Solid Edge part; units mm, degrees
sketch "Sketch1" plane through (0, 0, 0) normal (0, 0, 1) x (1, 0, 0)
  line L0 (-10, -20) -> (10, -20)
  line L1 (10, -20) -> (10, 20)
  line L2 (10, 20) -> (-10, 20)
  line L3 (-10, 20) -> (-10, -20)
extrude "Protrusion1" add sketch "Sketch1" along normal blind 62
sketch "Sketch2" plane through (-10, 0, 31) normal (-1, 0, 0) x (0, -1, 0)
  line L0 (20, -31) -> (20, -1)
  line L1 (20, -1) -> (1, -1)
  line L2 (1, -1) -> (1, -31)
  line L3 (1, -31) -> (20, -31)
  dimension "D1" = 1
extrude "Cutout1" cut sketch "Sketch2" along normal through all and the other way through all
sketch "Sketch3" plane through (-10, 0, 31) normal (-1, 0, 0) x (0, -1, 0)
  line L0 (-20, 31) -> (-8, 31)
  line L1 (-20, -7) -> (-8, 31)
  line L2 (-20, 31) -> (-20, -7)
extrude "Cutout2" cut sketch "Sketch3" along normal through all and the other way through all
hole "Hole1" at (7, 4, 62) direction (0, 0, -1) diameter 3 depth 9 tip angle 118
hole "Hole2" at (-7, 4, 62) direction (0, 0, -1) diameter 3 depth 9 tip angle 118
hole "Hole3" at (-7, -17, 62) direction (0, 0, -1) diameter 3 depth 9 tip angle 118
hole "Hole4" at (7, -17, 62) direction (0, 0, -1) diameter 3 depth 9 tip angle 118
sketch "Sketch4" plane through (0, -6, 62) normal (0, 0, 1) x (1, 0, 0)
  circle A0 centre (0, -4) radius 7
extrude "Cutout3" cut sketch "Sketch4" along normal up to next and the other way up to next
sketch "Sketch5" plane through (0, -20, 46) normal (0, -1, 0) x (1, 0, 0)
  circle A0 centre (-3, -1) radius 1.6
  circle A1 centre (3, -1) radius 1.6
  dimension "D1" = 3
extrude "Cutout4" cut sketch "Sketch5" along normal up to next and the other way up to next
sketch "Sketch6" plane through (0, 20, 12) normal (0, 1, 0) x (0, 0, -1)
  circle A0 centre (2, 0) radius 4
  dimension "D1" = 2
extrude "Cutout5" cut sketch "Sketch6" along normal up to next and the other way up to next
chamfer "Fase_an_schaft" distance 1 angle 45 1 edges at (0, 20, 14)
sketch "Sketch7" plane through (0, 9.5, 0) normal (0, 0, -1) x (1, 0, 0)
  circle A0 centre (0, 5.5) radius 2
extrude "Cutout6" cut sketch "Sketch7" along normal up to next and the other way up to next
hole "auslass_oben" at (0, 4, 62) direction (0, 0, -1) diameter 2.5 end up to next counterbore diameter 4 counterbore depth 30
sketch "Sketch8" plane through (-10, 0, 31) normal (-1, 0, 0) x (0, 0, -1)
  circle A0 centre (11, -12) radius 2.3428
extrude "Cutout7" cut sketch "Sketch8" along normal up to next and the other way up to next
sketch "Sketch9" plane through (0, 9.5, 0) normal (0, 0, -1) x (0, -1, 0)
  circle A0 centre (-2.5, 0) radius 2
extrude "auslassloch_hinten" cut sketch "Sketch9" against normal blind 20
sketch "Sketch10" plane through (0, -6, 62) normal (0, 0, 1) x (0, -1, 0)
  line L0 (-10, -2) -> (1.0843, -2)
  line L1 (1.0843, -2) -> (1.0843, 2)
  line L2 (1.0843, 2) -> (-10, 2)
  line L3 (-10, 2) -> (-10, -2)
  dimension "D1" = 1.0843
extrude "fräsung_oben" cut sketch "Sketch10" against normal blind 2
CAD build for the part. Positions are in the model's coordinates, mm. A direction names the side the tool comes from. Round coordinates to 2 decimals unless told otherwise and drop trailing zeros. Order: outer loops, then holes, each group sorted by start corner. A loop starts at its lowest first (then second) coordinate and runs counter-clockwise, first axis right, second up.
Item 1: Saw through at C-C on y = 12. Write the cut outline in (x, z).
Item 2: Tool access for faces 4 (the face through (-0.601, 10.092, 16.085)), 5 (the face through (-2, -17, 30)), 6 (the face through (-5.536, 4.325, 57.437)), 7 (the face through (-5.555, -14.259, 46.224)): list every direction of +Z, -Z, +X, -X, +Y, -Y with a clear straight run to the whole face (end or side of a thin tool).
Item 3: Saw through at B-B on z = 45. Write the cut outline in (x, y), then the cut area to 3 significant figures.
Item 4: Saw through at D-D on z = 17. Write the cut outline in (x, y), then the cut area to 3 significant figures.
Item 5: Probe line 1 along X through (y, z) = (-17.85, 45); line 2 along X through (y, z) = (12, 3.75); line 3 along X through (y, z) = (4, 27.25). List the from-to ranges inside material, lowest first.
Item 6: Mould opens along X. For faces 1 (the face through (0, 9, 14)), 2 (the face through (-0.1, 9.6, 0)), 3 (the face through (6.9, -17.241, 52.255)) say: pulls with the +X half, pulls with the -X half, needs draft (parallel to the pull), parting line crosses it, or undercut.
Item 7: Pin check, flat tips, straight feed: pin 1 (1.8 mm diameter, centred on x = -7, y = 4, fed in from +Z); pin 2 (3 mm diameter, centred on x = -3, z = 45, fed in from -Y); pin 3 (2.5 mm diameter, centred on x = 7, y = -17, fed in from -Z); pin 4 (5.5 mm diameter, centred on y = 12, z = 20, fed in from +X). Stop position of each tip, or through.
Item 8: Saw through at A-A on y = -4. Write the cut outline in (x, z), then the cut area to 3 significant figures.
Reported:
1. outline: (-10, 0) - (-2, 0) - (-2, 6.54) arc R4 cw to (-2, 13.46) - (-2, 17.66) - (-10, 17.66) - close; (-10, 22.34) - (10, 22.34) - (10, 49.33) - (-10, 49.33) - close; (2, 0) - (10, 0) - (10, 17.66) - (2, 17.66) - (2, 13.46) arc R4 cw to (2, 6.54) - close
2. face 4: -Z
2. face 5: -Z, +X, -X, -Y
2. face 6: +Z
2. face 7: +Z, -Z
3. outline: (-10, -20) - (-4.6, -20) - (-4.6, -15.28) arc R7 cw (long way) to (4.6, -15.28) - (4.6, -20) - (10, -20) - (10, 13.37) - (-10, 13.37) - close; (-1.4, -20) - (1.4, -20) - (1.4, -16.86) arc R7 cw to (-1.4, -16.86) - close; hole circle Ø4 at (0, 4)
3. area: 477 mm2
4. outline: (-10, -1) - (10, -1) - (10, 20) - (-10, 20) - close; hole circle Ø4 at (0, 12); hole circle Ø2.5 at (0, 4)
4. area: 403 mm2
5. line 1: x = -10 to -4.6, -1.4 to 1.4, 4.6 to 10
5. line 2: x = -10 to -2, 2 to 10
5. line 3: x = -10 to -1.25, 1.25 to 10
6. face 1: undercut
6. face 2: needs draft
6. face 3: undercut
7. pin 1: stops at z = 52.64
7. pin 2: stops at y = -4.64
7. pin 3: stops at z = 30
7. pin 4: stops at x = 10
8. outline: (-10, 30) - (-3.61, 30) - (-3.61, 62) - (-10, 62) - close; (3.61, 30) - (10, 30) - (10, 62) - (3.61, 62) - close
8. area: 409 mm2
